```python
from build123d import *

# Parameters (mm, degrees)
SKETCH_4_W          = 0.7
SKETCH_4_H          = 0.8
CUT_EXTRUDE_1_DEPTH = 50
SKETCH_6_R          = 4.963910668
CUT_EXTRUDE_2_DEPTH = 5
CHAMFER_1_SIZE      = 0.25


with BuildPart() as part:
    # 草图3 → Revolve 929 (revolve)
    with BuildSketch(Plane.XY, mode=Mode.PRIVATE) as revolve_929_sk:
        with BuildLine():
            Line((0, 0), (13.8, 0))
            Line((13.8, 0), (13.8, 1.5))
            Line((13.8, 1.5), (2.8, 1.5))
            Line((2.8, 1.5), (2.599, 1.299))
            Line((2.599, 1.299), (2.301, 1.299))
            ThreePointArc((2.301, 1.299), (1.946739503, 1.445739503), (1.8, 1.8))
            Line((1.8, 1.8), (1.8, 2.8))
            Line((1.8, 2.8), (0.821559832, 2.714397577))
            ThreePointArc((0.821559832, 2.714397577), (0.236450397, 2.425853536), (0, 1.817822349))
            Line((0, 1.817822349), (0, 0))
        make_face()
    revolve(revolve_929_sk.sketch.rotate(Axis((-2.477021524, 0, 0), (1, 0, 0)), 90), axis=Axis((-2.477021524, 0, 0), (1, 0, 0)))

    # 草图4 → 切除-拉伸1 (cut, symmetric)
    with BuildSketch(Plane.XY):
        with Locations((0.35, 0)):
            Rectangle(SKETCH_4_W, SKETCH_4_H)
    extrude(amount=CUT_EXTRUDE_1_DEPTH, both=True, mode=Mode.SUBTRACT)

    # 草图5 → 切除-旋转1 (revolve, cut)
    with BuildSketch(Plane.XY, mode=Mode.PRIVATE) as cut_revolve_1_sk:
        Polygon((13.547291997, 1.5), (14.047291997, 1.5), (13.8, 1.067), align=None)
    revolve(cut_revolve_1_sk.sketch.rotate(Axis((6.174994867, 0, 0), (-1, 0, 0)), 270), axis=Axis((6.174994867, 0, 0), (-1, 0, 0)), mode=Mode.SUBTRACT)

    # 草图6 → 切除-拉伸2 (cut)
    with BuildSketch(Plane(origin=(13.8, 0, 0), x_dir=(0, 0, -1), z_dir=(1, 0, 0))):
        Circle(SKETCH_6_R)
    extrude(amount=-CUT_EXTRUDE_2_DEPTH, mode=Mode.SUBTRACT)

    # 倒角1
    chamfer_1_edges = [part.edges().sort_by_distance(p)[0] for p in [
        (8.8, 0, -1.5),
    ]]
    chamfer(chamfer_1_edges, length=CHAMFER_1_SIZE)


solid = part.part
```
The listing builds one solid part. Answer for the finished solid, in the listing's coordinates (mm). A direction names the side the tool comes from. Give positions to 0.01 mm unless a question says otherwise; leave off trailing zeros. Order: outer loops, then holes, each group sorted by start corner. A loop starts at its lowest first (then second) coordinate and runs counter-clockwise, first axis right, second up.
Item 1: Find the intervals of material crossed by probe 1 along Y at (x, z) = (7.5, 0.05); probe 2 along X at (y, z) = (0.25, -1.9); probe 3 along X at (y, z) = (-1.4, -0.3), in increasing order.
From the geometry:
probe 1: y = -1.5 to 1.5
probe 2: x = 0.7 to 1.8
probe 3: x = 0 to 1.96, 2.73 to 8.62
Item 2: The part is cut by section B-B, the plane z = 0. Give the vertices of the cut face in (x, y), and give its area (3 significant figures).
From the geometry:
outline: (0, -1.82) arc R0.9 ccw to (0.82, -2.71) - (1.8, -2.8) - (1.8, -1.8) arc R0.5 cw to (2.3, -1.3) - (2.6, -1.3) - (2.8, -1.5) - (8.55, -1.5) - (8.8, -1.25) - (8.8, 1.25) - (8.55, 1.5) - (2.8, 1.5) - (2.6, 1.3) - (2.3, 1.3) arc R0.5 cw to (1.8, 1.8) - (1.8, 2.8) - (0.82, 2.71) arc R0.9 ccw to (0, 1.82) - (0, 0.4) - (0.7, 0.4) - (0.7, -0.4) - (0, -0.4) - close
area: 29.6 mm2
Item 3: Given pin 1 Ø0.8 at (x, z) = (0.5, 0) entering from -Y; pin 2 Ø0.6 at (x, z) = (0.5, 0.5) entering from +Y; pin 3 Ø0.6 at (y, z) = (0, 1) entering from -X, each flat-ended and moving along its own axis, determine where each tip first touches the part or whether it passes through.
From the geometry:
pin 1: stops at y = -2.72
pin 2: stops at y = 2.68
pin 3: stops at x = 0.7
Item 4: Which of the six approach directions +Z, -Z, +X, -X, +Y, -Y give full straight-line access (tool end or side, diameter ignored) to faces 1 (the face through (0.7, 0, 0)), 2 (the face through (5.63, -0.45, 1.43)), 3 (the face through (1.09, 1.67, -2.17))?
From the geometry:
face 1: +Z, -Z, -X
face 2: +X
face 3: -X
Item 5: The part is cut by section D-D, the plane x = 1. Give the vertices of the cut face in (y, z), and give its area (3 significant figures).
From the geometry:
outline: circle Ø5.46 at (0, 0)
area: 23.4 mm2
Item 6: The part is cut by section A-A, the plane y = 0. Give the vertices of the cut face in (x, z).
From the geometry:
outline: (0.7, -2.7) arc R0.9 ccw to (0.82, -2.71) - (1.8, -2.8) - (1.8, -1.8) arc R0.5 cw to (2.3, -1.3) - (2.6, -1.3) - (2.8, -1.5) - (8.55, -1.5) - (8.8, -1.25) - (8.8, 1.25) - (8.55, 1.5) - (2.8, 1.5) - (2.6, 1.3) - (2.3, 1.3) arc R0.5 cw to (1.8, 1.8) - (1.8, 2.8) - (0.82, 2.71) arc R0.9 ccw to (0.7, 2.7) - close
Item 7: The part is cut by section C-C, the plane x = 3.25. Give the vertices of the cut face in (y, z).
From the geometry:
outline: circle Ø3 at (0, 0)
